For this review, take the finished solid that the model builds, in its own axes (mm). A direction names the side the tool comes from. Coordinates: 2 decimals unless noted, no trailing zeros. Write each loop counter-clockwise with the first axis right and the second up, starting at its lowest first coordinate (ties: lowest second). Pieces come first, ordered by that corner, then holes.
1) We need section D-D on y = 4. Write out the cut boundary in (x, z) (3 decimals).
2) We need section A-A on z = -5. Write out the cut boundary in (x, y) (3 decimals), then the cut area to 3 significant figures.
3) Insertion check: P1, Ø6.5, axis at x = 25, z = -33.5, coming from the -Y side; P2, Ø5, axis at y = 7.5, z = 8.5, coming from the +X side; P3, Ø3.5, axis at x = 0.5, y = 37, coming from the +Z side; P4, Ø11.5, axis at x = 8, y = 18.5, coming from the -Z side (3 decimals). Each pin has a flat end and moves straight along its axis. Give the tip position at first contact, or say it passes through.
4) For faces 4 (the face through (0, 19, -19.05)), 5 (the face through (-27, 12.7, -29)), 6 (the face through (0, 36, 12.7)), 7 (the face through (-25.4, 19, -35)), 8 (the face through (19.05, 6, -25)), list the 3-axis set-ups (+Z, -Z, +X, -X, +Y, -Y) from which the entire face can be reached by the end or side of a thin tool; tool diameter is ignored.
5) We need section B-B on x = 11.5. Write out the cut boundary in (y, z) (3 decimals).
6) Mouldability with a two-part tool opening along X and no side actions: class faces 1 (the face through (25.4, 19, -35)), 2 (the face through (19.05, 32, -25)), 3 (the face through (0, 38.1, -3)) as pulls with the +X half, pulls with the -X half, needs draft (parallel to the pull), parting line crosses it, or undercut.
7) To check wall thickness, follow line 1 along Y through (x, z) = (-16, -18.5) (3 decimals); line 2 along X through (y, z) = (19, -33); line 3 along Z through (x, y) = (7, 22) (3 decimals). State the ranges of each line that lie inside material, in increasing order.
8) We need section C-C on z = 16. Write out the cut boundary in (x, y) (3 decimals).
Autodesk Fusion 360 part; units mm, degrees
sketch "Sketch1" plane through (0, 0, 0) normal (0, 1, 0) x (1, 0, 0)
  line L0 (19.05, 22.225) -> (-19.05, 22.225)
  line L1 (-19.05, 22.225) -> (-19.05, -22.225)
  line L2 (-19.05, -22.225) -> (19.05, -22.225)
  line L3 (19.05, -22.225) -> (19.05, 22.225)
  line L4 (0, -22.225) -> (12.7, -22.225)
  line L5 (0, -22.225) -> (-12.7, -22.225)
  line L6 (-19.05, 22.225) -> (-12.7, -22.225)
  line L7 (12.7, -22.225) -> (19.05, 22.225)
  line L8 (0, -22.225) -> (3.175, -22.225)
  line L9 (0, -22.225) -> (-3.175, -22.225)
  line L10 (-3.175, -22.225) -> (-3.175, -12.7)
  line L11 (3.175, -22.225) -> (3.175, -12.7)
  line L12 (-3.175, -12.7) -> (3.175, -12.7)
  dimension "d1" = 38.1
  dimension "d2" = 44.45
extrude "Extrude1" add sketch "Sketch1" along normal blind 38.1 contours L0 L2 L4 L5 L6 L7 L10 L11 L12 makes body 1
sketch "Sketch2" plane through (0, 0, 0) normal (0, -1, 0) x (1, 0, 0)
  line L0 (-3.175, 12.7) -> (-3.175, 22.225)
  line L1 (-3.175, 22.225) -> (-12.7, 22.225)
  line L2 (-12.7, 22.225) -> (-19.05, -22.225)
  line L3 (-19.05, -22.225) -> (19.05, -22.225)
  line L4 (19.05, -22.225) -> (12.7, 22.225)
  line L5 (12.7, 22.225) -> (3.175, 22.225)
  line L6 (3.175, 22.225) -> (3.175, 12.7)
  line L7 (3.175, 12.7) -> (-3.175, 12.7)
sketch "Sketch3" plane through (0, 0, 0) normal (1, 0, 0) x (0, 1, 0)
  line L0 (0, 0) -> (38.1, 0) construction
  line L1 (19.05, 0) -> (19.05, -22.225) construction
  line L2 (19.05, 0) -> (19.05, 22.225) construction
  line L3 (19.05, 22.225) -> (3.175, 22.225) construction
  line L4 (3.175, 22.225) -> (34.925, 22.225)
  line L5 (34.925, 22.225) -> (34.925, -19.05)
  line L6 (34.925, -19.05) -> (3.175, -19.05)
  line L7 (3.175, -19.05) -> (3.175, 22.225)
  dimension "d13" = 31.75
  dimension "d14" = 41.275
extrude "Extrude2" cut sketch "Sketch3" along normal blind 76.2 and the other way blind 60.96 bodies 1
extrude "Extrude3" add 1 faces at (6.35, 12.7, -22.225) along direction (0, 0, -1) blind 6.35 on bodies 1 bodies 1
sketch "Sketch4" plane through (19.05, 0, 0) normal (1, 0, 0) x (0, 1, 0)
  line L0 (38.1, -22.225) -> (0, -22.225)
  line L1 (0, -22.225) -> (0, -28.575)
  line L2 (0, -28.575) -> (38.1, -28.575)
  line L3 (38.1, -28.575) -> (38.1, -22.225)
  line L4 (19.05, -22.225) -> (25.4, -22.225)
  line L5 (19.05, -22.225) -> (12.7, -22.225)
  line L6 (12.7, -22.225) -> (12.7, -28.575)
  line L7 (25.4, -22.225) -> (25.4, -28.575)
  line L8 (12.7, -28.575) -> (25.4, -28.575)
  dimension "d21" = 6.35
extrude "Extrude4" add sketch "Sketch4" along normal blind 12.7 contours L0 L2 L4 L5 L6 L7 L8 bodies 1
extrude "Extrude5" add 1 faces at (31.75, 21.1667, -26.4583) along direction (-1, 0, 0) blind 63.5 on bodies 1 bodies 1
copy_body "Body->Comp1" bodies 1 removing the originals makes body 2 in component "Lower Anvil Holder"
sketch "Sketch5" plane through (0, 0, -28.575) normal (0, 0, -1) x (1, 0, 0)
  line L0 (19.05, -12.7) -> (19.05, 0)
  line L1 (19.05, 0) -> (-19.05, 0)
  line L2 (-19.05, 0) -> (-19.05, -12.7)
  line L3 (-19.05, -12.7) -> (-31.75, -12.7)
  line L4 (-31.75, -12.7) -> (-31.75, -25.4)
  line L5 (-31.75, -25.4) -> (-19.05, -25.4)
  line L6 (-19.05, -25.4) -> (-19.05, -38.1)
  line L7 (-19.05, -38.1) -> (19.05, -38.1)
  line L8 (19.05, -38.1) -> (19.05, -25.4)
  line L9 (19.05, -25.4) -> (31.75, -25.4)
  line L10 (31.75, -25.4) -> (31.75, -12.7)
  line L11 (31.75, -12.7) -> (19.05, -12.7)
  line L12 (31.75, -19.05) -> (25.4, -19.05) construction
  line L13 (25.4, -19.05) -> (25.4, -12.7)
  line L14 (25.4, -19.05) -> (25.4, -25.4)
  line L15 (-31.75, -19.05) -> (-25.4, -19.05) construction
  line L16 (-25.4, -19.05) -> (-25.4, -12.7)
  line L17 (-25.4, -19.05) -> (-25.4, -25.4)
  dimension "d27" = 6.35
  dimension "d28" = 6.35
extrude "Extrude1'" add sketch "Sketch5" along normal blind 12.7 contours L9 L10 L11 L13 L14 | L3 L4 L5 L16 L17 bodies 2 in component "Lower Anvil Holder"
fillet "Fillet1" radius 5.08 2 edges at (-31.75, 19.05, -22.225) (31.75, 19.05, -22.225) on bodies 2 in component "Lower Anvil Holder"
component "Lower Anvil Holder" placed x (1, 0, 0) y (0, 1, 0) z (0, 0, 1) at (0, 0, 0)
Result:
1. outline: (-19.05, -28.575) - (19.05, -28.575) - (19.05, -22.225) - (18.596, -19.05) - (-18.596, -19.05) - (-19.05, -22.225) - close
2. outline: (-16.589, 0) - (16.589, 0) - (16.589, 3.175) - (-16.589, 3.175) - close; (-16.589, 34.925) - (16.589, 34.925) - (16.589, 38.1) - (-16.589, 38.1) - close
2. area: 211 mm2
3. P1: stops at y = 12.7
3. P2: passes through
3. P3: stops at z = 12.7
3. P4: stops at z = -28.575
4. face 4: +Z, +X, -X
4. face 5: +Z, -Z, -X, -Y
4. face 6: +Z, +Y, -Y
4. face 7: -Z, +Y, -Y
4. face 8: +Z, -Z, +X, -Y
5. outline: (0, -28.575) - (38.1, -28.575) - (38.1, 22.225) - (34.925, 22.225) - (34.925, -19.05) - (3.175, -19.05) - (3.175, 22.225) - (0, 22.225) - close
6. face 1: undercut
6. face 2: pulls with the +X half
6. face 3: needs draft
7. line 1: y = 0 to 3.175, 34.925 to 38.1
7. line 2: x = -31.75 to -25.4, 25.4 to 31.75
7. line 3: z = -28.575 to -19.05
8. outline: (-13.589, 0) - (-3.175, 0) - (-3.175, 3.175) - (-13.589, 3.175) - close; (-13.589, 34.925) - (-3.175, 34.925) - (-3.175, 38.1) - (-13.589, 38.1) - close; (3.175, 0) - (13.589, 0) - (13.589, 3.175) - (3.175, 3.175) - close; (3.175, 34.925) - (13.589, 34.925) - (13.589, 38.1) - (3.175, 38.1) - close
